Here's the drawing with two shaded views (mm, measured from the low corner). I have some questions. A direction names the side the tool comes from. Give positions to 0.01 mm unless a question says otherwise; leave off trailing zeros. Write each loop counter-clockwise with the first axis right and the second up, starting at its lowest first coordinate (ties: lowest second). Pieces come first, ordered by that corner, then holes. Notation, with made-up numbers: (38.5, -35.75) - (69.5, -35.75) arc R20 ccw to (69.5, -31.75) - close; hole circle Ø4 at (71.5, 87). An arc over 180 degrees is marked (long way). Write item = value, one per line.
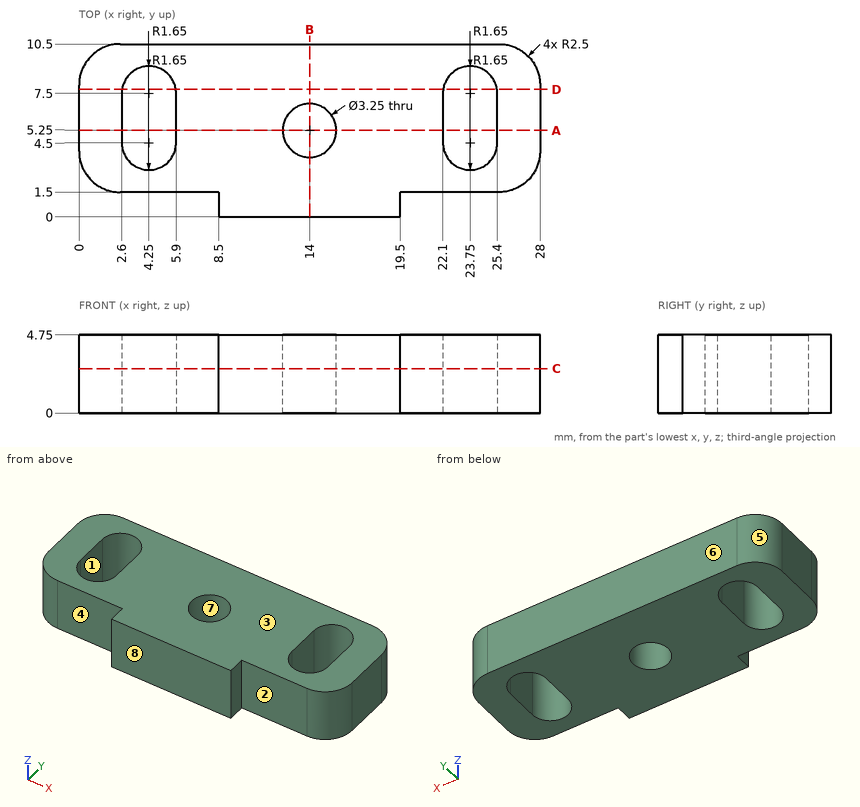
1. If we section it at C-C, the plane z = 2.7: Please give me the cut outline in (x, y) (3 decimals), and give its area (3 significant figures).
Filled sheet:
outline = (0, 4) arc R2.5 ccw to (2.5, 1.5) - (8.5, 1.5) - (8.5, 0) - (19.5, 0) - (19.5, 1.5) - (25.5, 1.5) arc R2.5 ccw to (28, 4) - (28, 8) arc R2.5 ccw to (25.5, 10.5) - (2.5, 10.5) arc R2.5 ccw to (0, 8) - close; hole (2.6, 4.5) arc R1.65 ccw to (5.9, 4.5) - (5.9, 7.5) arc R1.65 ccw to (2.6, 7.5) - close; hole circle Ø3.25 at (14, 5.25); hole (22.1, 4.5) arc R1.65 ccw to (25.4, 4.5) - (25.4, 7.5) arc R1.65 ccw to (22.1, 7.5) - close
area = 218 mm2
2. If we section it at A-A, the plane y = 5.25: Please give me the cut outline in (x, z) (3 decimals), and give its area (3 significant figures).
Filled sheet:
outline = (0, 0) - (2.6, 0) - (2.6, 4.75) - (0, 4.75) - close; (5.9, 0) - (12.375, 0) - (12.375, 4.75) - (5.9, 4.75) - close; (15.625, 0) - (22.1, 0) - (22.1, 4.75) - (15.625, 4.75) - close; (25.4, 0) - (28, 0) - (28, 4.75) - (25.4, 4.75) - close
area = 86.2 mm2
3. I need wall thicknesses on line 1 (X direction, y = 5.25, z = 1.9) (3 decimals); line 2 (Y direction, x = 14, z = 1.05) (3 decimals); line 3 (X direction, y = 4, z = 1.4). Which ranges of each line are inside material? Lowest first, please.
Filled sheet:
line_1 = 0 to 2.6, 5.9 to 12.375, 15.625 to 22.1, 25.4 to 28
line_2 = 0 to 3.625, 6.875 to 10.5
line_3 = 0 to 2.68, 5.82 to 12.96, 15.04 to 22.18, 25.32 to 28
4. Which directions (+Z, -Z, +X, -X, +Y, -Y) give clear straight access to the entire face, cutting with the end or side of a thin tool? Please do the marked faces 1, 2, 3, 4 and 5.
Filled sheet:
face_1 = +Z, -Z
face_2 = +Z, -Z, +X, -Y
face_3 = +Z, +X, -X, +Y, -Y
face_4 = +Z, -Z, -X, -Y
face_5 = +Z, -Z, -X, +Y
5. If we section it at B-B, the plane x = 14: Please give me the cut outline in (y, z) (3 decimals), and give its area (3 significant figures).
Filled sheet:
outline = (0, 0) - (3.625, 0) - (3.625, 4.75) - (0, 4.75) - close; (6.875, 0) - (10.5, 0) - (10.5, 4.75) - (6.875, 4.75) - close
area = 34.4 mm2
6. If we section it at D-D, the plane y = 7.75: Please give me the cut outline in (x, z).
Filled sheet:
outline = (0, 0) - (2.62, 0) - (2.62, 4.75) - (0, 4.75) - close; (5.88, 0) - (22.12, 0) - (22.12, 4.75) - (5.88, 4.75) - close; (25.38, 0) - (28, 0) - (28, 4.75) - (25.38, 4.75) - close
7. For pin 1 (1.4 mm diameter, centred on x = 23, z = 2.5, fed in from -Y); pin 2 (0.8 mm diameter, centred on y = 1, z = 2, fed in from -X), each with a flat end and sliding along its axis, tell me the tip position at first contact or that it passes through.
Filled sheet:
pin_1 = 1.5
pin_2 = 8.5
8. Thinking about a two-plate mould opening in Y: for the marked faces 6, 7 and 8, which applies, pulls with the +Y half, pulls with the -Y half, needs draft (parallel to the pull), parting line crosses it, or undercut?
Filled sheet:
face_6 = pulls with the +Y half
face_7 = undercut
face_8 = pulls with the -Y half
